Can you work these out from the model? Positions are in its coordinate system, mm. A direction names the side the tool comes from. Give positions to 0.01 mm unless a question says otherwise; leave off trailing zeros. Write each loop counter-clockwise with the first axis right and the second up, starting at its lowest first coordinate (ties: lowest second). Pieces come first, ordered by that corner, then holes. Notation, with made-up numbers: (-36, 46.25) -> (8, 46.25) arc R33 cw to (8, 78.25) -> close; hole circle Ø6 at (25.5, -25.75). An arc over 180 degrees is marked (long way). One line per item, written item: value.
from build123d import *

# Parameters (mm, degrees)
BOSS_EXTRUDE1_DEPTH = 2.5
BOSS_EXTRUDE2_DEPTH = 5
SKETCH4_W           = 60
SKETCH4_H           = 68
CUT_EXTRUDE1_DEPTH  = 5
SKETCH6_W           = 66
SKETCH6_H           = 74
SKETCH6_W_2         = 60
SKETCH6_H_2         = 68
BOSS_EXTRUDE3_DEPTH = 4
SKETCH7_R           = 1.65
CUT_EXTRUDE3_DEPTH  = 2.5


with BuildPart() as part:
    # Sketch1 → Boss-Extrude1 (new body)
    # profile 1 of 2: a face of its own
    with BuildSketch(Plane(origin=(0, 0, 0), x_dir=(1, 0, 0), z_dir=(0, 1, 0))):
        with BuildLine():
            ThreePointArc((-80, -96), (-92.02081528, -91.02081528), (-97, -79))
            Line((-97, -79), (-97, 79))
            ThreePointArc((-97, 79), (-92.02081528, 91.02081528), (-80, 96))
            Line((-80, 96), (80, 96))
            ThreePointArc((80, 96), (92.02081528, 91.02081528), (97, 79))
            Line((97, 79), (97, -79))
            ThreePointArc((97, -79), (92.02081528, -91.02081528), (80, -96))
            Line((80, -96), (-80, -96))
        make_face()
        with BuildLine():
            Line((-95, -79), (-95, 79))
            ThreePointArc((-95, 79), (-90.606601718, 89.606601718), (-80, 94))
            Line((-80, 94), (80, 94))
            ThreePointArc((80, 94), (90.606601718, 89.606601718), (95, 79))
            Line((95, 79), (95, -79))
            ThreePointArc((95, -79), (90.606601718, -89.606601718), (80, -94))
            Line((80, -94), (-80, -94))
            ThreePointArc((-80, -94), (-90.606601718, -89.606601718), (-95, -79))
        make_face(mode=Mode.SUBTRACT)
    # profile 2 of 2: a face of its own
    with BuildSketch(Plane(origin=(0, 0, 0), x_dir=(1, 0, 0), z_dir=(0, 1, 0))):
        with BuildLine():
            ThreePointArc((-95, 79), (-90.606601718, 89.606601718), (-80, 94))
            Line((-80, 94), (80, 94))
            ThreePointArc((80, 94), (90.606601718, 89.606601718), (95, 79))
            Line((95, 79), (95, -79))
            ThreePointArc((95, -79), (90.606601718, -89.606601718), (80, -94))
            Line((80, -94), (-80, -94))
            ThreePointArc((-80, -94), (-90.606601718, -89.606601718), (-95, -79))
            Line((-95, -79), (-95, 79))
        make_face()
    extrude(amount=BOSS_EXTRUDE1_DEPTH)

    # Sketch3 → Boss-Extrude2 (add)
    # profile 1 of 2: a face of its own
    with BuildSketch(Plane(origin=(0, 2.5, 0), x_dir=(1, 0, 0), z_dir=(0, 1, 0))):
        with BuildLine():
            Line((-97, 79), (-97, -79))
            ThreePointArc((-97, -79), (-92.02081528, -91.02081528), (-80, -96))
            Line((-80, -96), (80, -96))
            ThreePointArc((80, -96), (92.02081528, -91.02081528), (97, -79))
            Line((97, -79), (97, 79))
            ThreePointArc((97, 79), (92.02081528, 91.02081528), (80, 96))
            Line((80, 96), (-80, 96))
            ThreePointArc((-80, 96), (-92.02081528, 91.02081528), (-97, 79))
        make_face()
        with BuildLine():
            ThreePointArc((-95.2, -79), (-90.748023074, -89.748023074), (-80, -94.2))
            Line((-80, -94.2), (80, -94.2))
            ThreePointArc((80, -94.2), (90.748023074, -89.748023074), (95.2, -79))
            Line((95.2, -79), (95.2, 79))
            ThreePointArc((95.2, 79), (90.748023074, 89.748023074), (80, 94.2))
            Line((80, 94.2), (-80, 94.2))
            ThreePointArc((-80, 94.2), (-90.748023074, 89.748023074), (-95.2, 79))
            Line((-95.2, 79), (-95.2, -79))
        make_face(mode=Mode.SUBTRACT)
    # profile 2 of 2: a face of its own
    with BuildSketch(Plane(origin=(0, 2.5, 0), x_dir=(1, 0, 0), z_dir=(0, 1, 0))):
        with BuildLine():
            Line((-91.8, 79), (-91.8, -79))
            ThreePointArc((-91.8, -79), (-88.343860018, -87.343860018), (-80, -90.8))
            Line((-80, -90.8), (80, -90.8))
            ThreePointArc((80, -90.8), (88.343860018, -87.343860018), (91.8, -79))
            Line((91.8, -79), (91.8, 79))
            ThreePointArc((91.8, 79), (88.343860018, 87.343860018), (80, 90.8))
            Line((80, 90.8), (-80, 90.8))
            ThreePointArc((-80, 90.8), (-88.343860018, 87.343860018), (-91.8, 79))
        make_face()
        with BuildLine():
            ThreePointArc((-80, 89.3), (-87.283199846, 86.283199846), (-90.3, 79))
            Line((-90.3, 79), (-90.3, -79))
            ThreePointArc((-90.3, -79), (-87.283199846, -86.283199846), (-80, -89.3))
            Line((-80, -89.3), (80, -89.3))
            ThreePointArc((80, -89.3), (87.283199846, -86.283199846), (90.3, -79))
            Line((90.3, -79), (90.3, 79))
            ThreePointArc((90.3, 79), (87.283199846, 86.283199846), (80, 89.3))
            Line((80, 89.3), (-80, 89.3))
        make_face(mode=Mode.SUBTRACT)
    extrude(amount=BOSS_EXTRUDE2_DEPTH)

    # Sketch4 → Cut-Extrude1 (cut)
    with BuildSketch(Plane(origin=(0, 2.5, 0), x_dir=(1, 0, 0), z_dir=(0, 1, 0))):
        Rectangle(SKETCH4_W, SKETCH4_H)
    extrude(amount=-CUT_EXTRUDE1_DEPTH, mode=Mode.SUBTRACT)

    # Sketch6 → Boss-Extrude3 (add)
    with BuildSketch(Plane(origin=(0, 2.5, 0), x_dir=(1, 0, 0), z_dir=(0, 1, 0))):
        Rectangle(SKETCH6_W, SKETCH6_H)
        Rectangle(SKETCH6_W_2, SKETCH6_H_2, mode=Mode.SUBTRACT)
    extrude(amount=BOSS_EXTRUDE3_DEPTH)

    # Sketch7 → Cut-Extrude3 (cut)
    with BuildSketch(Plane(origin=(0, 2.5, 0), x_dir=(1, 0, 0), z_dir=(0, 1, 0))):
        with Locations(Location((-84.834554705, 15, 0), (0, 0, 270))):
            Circle(SKETCH7_R)
        with Locations(Location((-73.834554705, 15, 0), (0, 0, 270))):
            Circle(SKETCH7_R)
        with Locations(Location((-62.834554705, 15, 0), (0, 0, 270))):
            Circle(SKETCH7_R)
        with Locations(Location((-51.834554705, 15, 0), (0, 0, 270))):
            Circle(SKETCH7_R)
        with Locations(Location((-40.834554705, 15, 0), (0, 0, 270))):
            Circle(SKETCH7_R)
        with Locations(Location((-40.834554705, 0, 0), (0, 0, 270))):
            Circle(SKETCH7_R)
        with Locations(Location((-51.834554705, 0, 0), (0, 0, 270))):
            Circle(SKETCH7_R)
        with Locations(Location((-62.834554705, 0, 0), (0, 0, 270))):
            Circle(SKETCH7_R)
        with Locations(Location((-73.834554705, 0, 0), (0, 0, 270))):
            Circle(SKETCH7_R)
        with Locations(Location((-84.834554705, 0, 0), (0, 0, 270))):
            Circle(SKETCH7_R)
        with Locations(Location((-84.834554705, -15, 0), (0, 0, 270))):
            Circle(SKETCH7_R)
        with Locations(Location((-73.834554705, -15, 0), (0, 0, 270))):
            Circle(SKETCH7_R)
        with Locations(Location((-62.834554705, -15, 0), (0, 0, 270))):
            Circle(SKETCH7_R)
        with Locations(Location((-51.834554705, -15, 0), (0, 0, 270))):
            Circle(SKETCH7_R)
        with Locations(Location((-40.834554705, -15, 0), (0, 0, 270))):
            Circle(SKETCH7_R)
        with Locations(Location((15, 84.834554705, 0), (0, 0, 270))):
            Circle(SKETCH7_R)
        with Locations(Location((15, 73.834554705, 0), (0, 0, 270))):
            Circle(SKETCH7_R)
        with Locations(Location((15, 62.834554705, 0), (0, 0, 270))):
            Circle(SKETCH7_R)
        with Locations(Location((15, 51.834554705, 0), (0, 0, 270))):
            Circle(SKETCH7_R)
        with Locations(Location((15, 40.834554705, 0), (0, 0, 270))):
            Circle(SKETCH7_R)
        with Locations(Location((0, 40.834554705, 0), (0, 0, 270))):
            Circle(SKETCH7_R)
        with Locations(Location((0, 51.834554705, 0), (0, 0, 270))):
            Circle(SKETCH7_R)
        with Locations(Location((0, 62.834554705, 0), (0, 0, 270))):
            Circle(SKETCH7_R)
        with Locations(Location((0, 73.834554705, 0), (0, 0, 270))):
            Circle(SKETCH7_R)
        with Locations(Location((0, 84.834554705, 0), (0, 0, 270))):
            Circle(SKETCH7_R)
        with Locations(Location((-15, 84.834554705, 0), (0, 0, 270))):
            Circle(SKETCH7_R)
        with Locations(Location((-15, 73.834554705, 0), (0, 0, 270))):
            Circle(SKETCH7_R)
        with Locations(Location((-15, 62.834554705, 0), (0, 0, 270))):
            Circle(SKETCH7_R)
        with Locations(Location((-15, 51.834554705, 0), (0, 0, 270))):
            Circle(SKETCH7_R)
        with Locations(Location((-15, 40.834554705, 0), (0, 0, 270))):
            Circle(SKETCH7_R)
        with Locations(Location((84.834554705, -15, 0), (0, 0, 270))):
            Circle(SKETCH7_R)
        with Locations(Location((73.834554705, -15, 0), (0, 0, 270))):
            Circle(SKETCH7_R)
        with Locations(Location((62.834554705, -15, 0), (0, 0, 270))):
            Circle(SKETCH7_R)
        with Locations(Location((51.834554705, -15, 0), (0, 0, 270))):
            Circle(SKETCH7_R)
        with Locations(Location((40.834554705, -15, 0), (0, 0, 270))):
            Circle(SKETCH7_R)
        with Locations(Location((40.834554705, 0, 0), (0, 0, 270))):
            Circle(SKETCH7_R)
        with Locations(Location((51.834554705, 0, 0), (0, 0, 270))):
            Circle(SKETCH7_R)
        with Locations(Location((62.834554705, 0, 0), (0, 0, 270))):
            Circle(SKETCH7_R)
        with Locations(Location((73.834554705, 0, 0), (0, 0, 270))):
            Circle(SKETCH7_R)
        with Locations(Location((84.834554705, 0, 0), (0, 0, 270))):
            Circle(SKETCH7_R)
        with Locations(Location((84.834554705, 15, 0), (0, 0, 270))):
            Circle(SKETCH7_R)
        with Locations(Location((73.834554705, 15, 0), (0, 0, 270))):
            Circle(SKETCH7_R)
        with Locations(Location((62.834554705, 15, 0), (0, 0, 270))):
            Circle(SKETCH7_R)
        with Locations(Location((51.834554705, 15, 0), (0, 0, 270))):
            Circle(SKETCH7_R)
        with Locations(Location((40.834554705, 15, 0), (0, 0, 270))):
            Circle(SKETCH7_R)
        with Locations(Location((-15, -84.834554705, 0), (0, 0, 270))):
            Circle(SKETCH7_R)
        with Locations(Location((-15, -73.834554705, 0), (0, 0, 270))):
            Circle(SKETCH7_R)
        with Locations(Location((-15, -62.834554705, 0), (0, 0, 270))):
            Circle(SKETCH7_R)
        with Locations(Location((-15, -51.834554705, 0), (0, 0, 270))):
            Circle(SKETCH7_R)
        with Locations(Location((-15, -40.834554705, 0), (0, 0, 270))):
            Circle(SKETCH7_R)
        with Locations(Location((0, -40.834554705, 0), (0, 0, 270))):
            Circle(SKETCH7_R)
        with Locations(Location((0, -51.834554705, 0), (0, 0, 270))):
            Circle(SKETCH7_R)
        with Locations(Location((0, -62.834554705, 0), (0, 0, 270))):
            Circle(SKETCH7_R)
        with Locations(Location((0, -73.834554705, 0), (0, 0, 270))):
            Circle(SKETCH7_R)
        with Locations(Location((0, -84.834554705, 0), (0, 0, 270))):
            Circle(SKETCH7_R)
        with Locations(Location((15, -84.834554705, 0), (0, 0, 270))):
            Circle(SKETCH7_R)
        with Locations(Location((15, -73.834554705, 0), (0, 0, 270))):
            Circle(SKETCH7_R)
        with Locations(Location((15, -62.834554705, 0), (0, 0, 270))):
            Circle(SKETCH7_R)
        with Locations(Location((15, -51.834554705, 0), (0, 0, 270))):
            Circle(SKETCH7_R)
        with Locations(Location((15, -40.834554705, 0), (0, 0, 270))):
            Circle(SKETCH7_R)
    extrude(amount=-CUT_EXTRUDE3_DEPTH, mode=Mode.SUBTRACT)


solid = part.part
1) I need wall thicknesses on L1, parallel to X at y = 4.25, z = 51; L2, parallel to Z at x = -1, y = 6.25; L3, parallel to Z at x = -43.5, y = 6.75. Which ranges of each line are inside material? Lowest first, please.
Answer list:
L1: x = -97 to -95.2, -91.8 to -90.3, 90.3 to 91.8, 95.2 to 97
L2: z = -96 to -94.2, -90.8 to -89.3, -37 to -34, 34 to 37, 89.3 to 90.8, 94.2 to 96
L3: z = -96 to -94.2, -90.8 to -89.3, 89.3 to 90.8, 94.2 to 96
2) We'd pull the mould along X, two halves only. Please class faces 4 (the face through (1, 0, -44)), 5 (the face through (87.203, 4.965, 86.363)), 6 (the face through (91.89, 3.7, 91.15)), 7 (the face through (1, 5, -94.2)): released by +X, released by -X, zero draft, split by the parting line, or undercut.
Answer list:
face 4: zero draft
face 5: undercut
face 6: released by +X
face 7: undercut
3) Will this pin go through, and if not, where does the flat tip stop? pin 1 (5.5 mm diameter, centred on x = 15, z = -84.83, fed in from +Y).
Answer list:
pin 1: stops at y = 2.5
4) If we section it at B-B (x = -20): Write out the boundary of the cut face in (y, z), and give its area (3 significant figures).
Answer list:
outline: (0, -96) -> (7.5, -96) -> (7.5, -94.2) -> (2.5, -94.2) -> (2.5, -90.8) -> (7.5, -90.8) -> (7.5, -89.3) -> (2.5, -89.3) -> (2.5, -37) -> (6.5, -37) -> (6.5, -34) -> (0, -34) -> close; (0, 34) -> (6.5, 34) -> (6.5, 37) -> (2.5, 37) -> (2.5, 89.3) -> (7.5, 89.3) -> (7.5, 90.8) -> (2.5, 90.8) -> (2.5, 94.2) -> (7.5, 94.2) -> (7.5, 96) -> (0, 96) -> close
area: 367 mm^2
5) If we section it at A-A (z = -21): Write out the boundary of the cut face in (x, y), and give its area (3 significant figures).
Answer list:
outline: (-97, 0) -> (-30, 0) -> (-30, 6.5) -> (-33, 6.5) -> (-33, 2.5) -> (-90.3, 2.5) -> (-90.3, 7.5) -> (-91.8, 7.5) -> (-91.8, 2.5) -> (-95.2, 2.5) -> (-95.2, 7.5) -> (-97, 7.5) -> close; (30, 0) -> (97, 0) -> (97, 7.5) -> (95.2, 7.5) -> (95.2, 2.5) -> (91.8, 2.5) -> (91.8, 7.5) -> (90.3, 7.5) -> (90.3, 2.5) -> (33, 2.5) -> (33, 6.5) -> (30, 6.5) -> close
area: 392 mm^2
6) For faces 1 (the face through (-91.89, 3.7, -91.15)), 2 (the face through (30, 3, 0)), 3 (the face through (88.252, 4.965, 87.435)), which set-ups out of +Z, -Z, +X, -X, +Y, -Y let a thin tool reach every point of the face, with its end or its side?
Answer list:
face 1: -Z, -X, +Y, -Y
face 2: +Y, -Y
face 3: +Y
7) If we section it at C-C (z = -67.5): Write out the boundary of the cut face in (x, y).
Answer list:
outline: (-97, 0) -> (97, 0) -> (97, 7.5) -> (95.2, 7.5) -> (95.2, 2.5) -> (91.8, 2.5) -> (91.8, 7.5) -> (90.3, 7.5) -> (90.3, 2.5) -> (-90.3, 2.5) -> (-90.3, 7.5) -> (-91.8, 7.5) -> (-91.8, 2.5) -> (-95.2, 2.5) -> (-95.2, 7.5) -> (-97, 7.5) -> close
8) If we section it at D-D (x = -56): Write out the boundary of the cut face in (y, z), and give its area (3 significant figures).
Answer list:
outline: (0, -96) -> (7.5, -96) -> (7.5, -94.2) -> (2.5, -94.2) -> (2.5, -90.8) -> (7.5, -90.8) -> (7.5, -89.3) -> (2.5, -89.3) -> (2.5, 89.3) -> (7.5, 89.3) -> (7.5, 90.8) -> (2.5, 90.8) -> (2.5, 94.2) -> (7.5, 94.2) -> (7.5, 96) -> (0, 96) -> close
area: 513 mm^2
